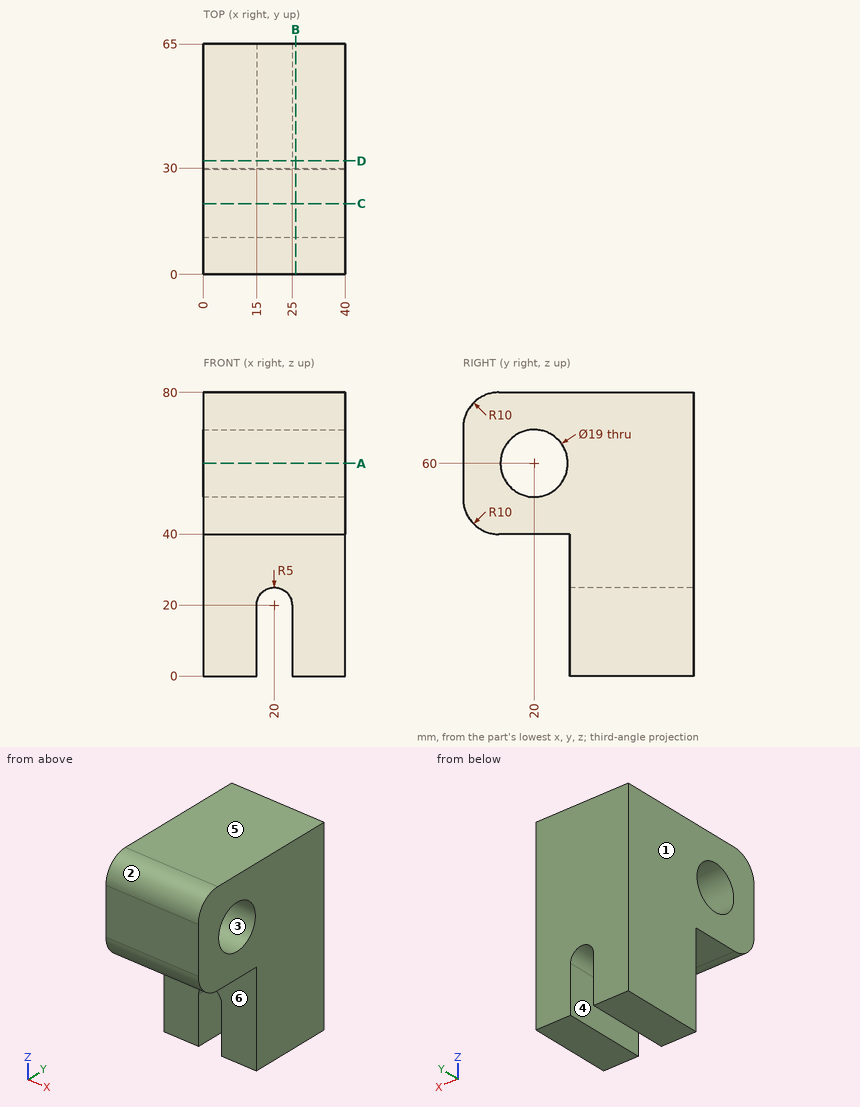
Study the drawing (mm; zero at the part's minimum x, y, z) and answer. A direction names the side the tool comes from. Round coordinates to 2 decimals unless told otherwise and drop trailing zeros. Write each loop counter-clockwise with the first axis right and the second up, starting at its lowest first coordinate (ties: lowest second). Pieces come first, ordered by that corner, then holes.
Q1. Flat-ended cylindrical pins translate along their axes: P1, Ø20, axis at x = 26, z = 19, coming from the -Y side; P2, Ø6, axis at x = 13.5, y = 20, coming from the -Z side; P3, Ø5, axis at x = 35, z = 39, coming from the -Y side; P4, Ø5, axis at y = 25.5, z = 29.5, coming from the -X side. Find the tip coordinate at first contact, or state that the pin passes through.
Values:
P1: stops at y = 30
P2: stops at z = 40
P3: stops at y = 4.73
P4: passes through
Q2. Find section A-A on z = 60. Determine the outline of the cut face in (x, y), and give its area (3 significant figures).
Values:
outline: (0, 0) - (40, 0) - (40, 10.5) - (0, 10.5) - close; (0, 29.5) - (40, 29.5) - (40, 65) - (0, 65) - close
area: 1,840 mm2
Q3. Find section D-D on y = 32. Determine the outline of the cut face in (x, z), and give its area (3 significant figures).
Values:
outline: (0, 0) - (15, 0) - (15, 20) arc R5 cw to (25, 20) - (25, 0) - (40, 0) - (40, 80) - (0, 80) - close
area: 2,960 mm2
Q4. A tool of negligible diameter and unlimited length cuts with its end or side. For the marked faces 4, 5 and 6, from which of +Z, -Z, +X, -X, +Y, -Y can it reach the whole face along a straight path? Write none if from no direction.
Values:
face 4: -Z, +Y, -Y
face 5: +Z, +X, -X, +Y, -Y
face 6: -Z, +X, -X, -Y
Q5. Straight lines are drawn through the part: line 1 (Z direction, x = 15, y = 20); line 2 (Y direction, x = 31.5, z = 59.5); line 3 (X direction, y = 59.5, z = 18.5). For each, find the intervals that lie inside material, in ascending order.
Values:
line 1: z = 40 to 50.5, 69.5 to 80
line 2: y = 0 to 10.51, 29.49 to 65
line 3: x = 0 to 15, 25 to 40
Q6. The mould has two halves that part along Y. Classify the marked faces 1, 2 and 3: released by +Y, released by -Y, zero draft, split by the parting line, or undercut.
Values:
face 1: zero draft
face 2: released by -Y
face 3: undercut
Q7. Find section B-B on x = 26. Determine the outline of the cut face in (y, z), and give its area (3 significant figures).
Values:
outline: (0, 50) arc R10 ccw to (10, 40) - (30, 40) - (30, 0) - (65, 0) - (65, 80) - (10, 80) arc R10 ccw to (0, 70) - close; hole circle Ø19 at (20, 60)
area: 3,670 mm2
Q8. Find section C-C on y = 20. Determine the outline of the cut face in (x, z), and give its area (3 significant figures).
Values:
outline: (0, 40) - (40, 40) - (40, 50.5) - (0, 50.5) - close; (0, 69.5) - (40, 69.5) - (40, 80) - (0, 80) - close
area: 840 mm2
